from build123d import *

# Parameters (mm, degrees)
F1_DEPTH = 15


with BuildPart() as f1:
    # F0 (on Top) → F1 (new body)
    with BuildSketch(Plane.XY):
        with BuildLine():
            Line((0, 150), (0, 0))
            Line((0, 0), (21.132487, 0))
            Line((21.132487, 0), (36.03576, 25.813227))
            ThreePointArc((36.03576, 25.813227), (36.252826, 27.261495), (35.424873, 28.469425))
            ThreePointArc((35.424873, 28.469425), (50, 76), (64.575127, 28.469425))
            ThreePointArc((64.575127, 28.469425), (63.747174, 27.261495), (63.96424, 25.813227))
            Line((63.96424, 25.813227), (78.867513, 0))
            Line((78.867513, 0), (100, 0))
            Line((100, 0), (100, 150))
            Line((100, 150), (0, 150))
        make_face()
    extrude(amount=F1_DEPTH)


solid = f1.part
Verification items for the finished model (mm, model axes). A direction names the side the tool comes from. Give positions to 0.01 mm unless a question says otherwise; leave off trailing zeros. Write each loop counter-clockwise with the first axis right and the second up, starting at its lowest first coordinate (ties: lowest second). Pieces come first, ordered by that corner, then holes. Notation, with made-up numbers: M 80,67.25 L 107,67.25 A21 cw 107,105.25 Z; hole C 42.25,68 d5. An arc over 180 degrees is marked long. Use CSV: the item, a comma, the result in double quotes.
1) Go/stop test with flat-tipped pins: pin 1 Ø3 at (y, z) = (53.5, 12) entering from -X; pin 2 Ø8 at (x, z) = (55.5, 11.5) entering from -Y. Record where each tip stops, or that it passes through.
Final values:
pin 1,"x = 0"
pin 2,"y = 74.2"
2) Access from +Z, -Z, +X, -X, +Y, -Y to the whole of each face (thin tool, end or side, straight path). Record for faces 4 (the face through (49, 93, 15)), 5 (the face through (28.48, 12.73, 7.4)).
Final values:
face 4,"+Z, +X, -X, +Y, -Y"
face 5,"+Z, -Z, -Y"
3) Material ranges on line 1 along X through (y, z) = (50, 3.75); line 2 along Y through (x, z) = (66.5, 11.5); line 3 along Y through (x, z) = (35, 10.75), recorded low to high.
Final values:
line 1,"0 to 24, 76 to 100"
line 2,"21.42 to 29.91, 70.09 to 150"
line 3,"24.02 to 28.76, 71.24 to 150"
4) Release check for a two-part mould opening along X. For faces 1 (the face through (10, 0, 7)), 2 (the face through (100, 74, 7)), 3 (the face through (71.31, 13.09, 7.4)) record: released by +X, released by -X, zero draft, split by the parting line, or undercut.
Final values:
face 1,"zero draft"
face 2,"released by +X"
face 3,"undercut"
5) Cross-section at A-A (y = 50). Enter the section's corners in (x, z).
Final values:
outline,"M 0,0 L 24,0 L 24,15 L 0,15 Z; M 76,0 L 100,0 L 100,15 L 76,15 Z"
6) Cross-section at D-D (x = 50). Enter the section's corners in (y, z).
Final values:
outline,"M 76,0 L 150,0 L 150,15 L 76,15 Z"
7) Cross-section at C-C (z = 9). Enter the section's corners in (x, y), plus the area to 3 significant figures.
Final values:
outline,"M 0,0 L 21.13,0 L 36.04,25.81 A2 ccw 35.42,28.47 A26 cw long 64.58,28.47 A2 ccw 63.96,25.81 L 78.87,0 L 100,0 L 100,150 L 0,150 Z"
area,"11,800 mm²"
8) Cross-section at B-B (x = 70). Enter the section's corners in (y, z).
Final values:
outline,"M 15.36,0 L 33.39,0 L 33.39,15 L 15.36,15 Z; M 66.61,0 L 150,0 L 150,15 L 66.61,15 Z"
